```python
from build123d import *

# Parameters (mm, degrees)
SKETCH1_W            = 76
SKETCH1_H            = 41
BOSS_EXTRUDE1_DEPTH  = 1
SKETCH2_W            = 9
SKETCH2_H            = 9
BOSS_EXTRUDE2_DEPTH  = 1
SKETCH3_R            = 1.6
CUT_EXTRUDE1_DEPTH   = 1
FILLET1_R            = 1
FILLET3_R            = 3
FILLET1_OF_MIRROR2_R = 1
MIRROR3_OUTLINE_R    = 1.6
MIRROR3_DEPTH        = 1
FILLET4_R            = 3


# Read off the part's stored shape, not the designer's step: Mirror3
with BuildPart() as part:
    # Sketch1 → Boss-Extrude1 (new body)
    with BuildSketch(Plane(origin=(0, 0, 0), x_dir=(1, 0, 0), z_dir=(0, 1, 0))):
        Rectangle(SKETCH1_W, SKETCH1_H)
    boss_extrude1 = extrude(amount=BOSS_EXTRUDE1_DEPTH)

    # Sketch2 → Boss-Extrude2 (add)
    with BuildSketch(Plane(origin=(0, 1, 0), x_dir=(1, 0, 0), z_dir=(0, 1, 0))):
        with Locations((40.5, 23)):
            Rectangle(SKETCH2_W, SKETCH2_H)
    boss_extrude2 = extrude(amount=-BOSS_EXTRUDE2_DEPTH)

    # Sketch3 → Cut-Extrude1 (cut)
    with BuildSketch(Plane(origin=(0, 1, 0), x_dir=(1, 0, 0), z_dir=(0, 1, 0))):
        with Locations(Location((40.5, 22.887482194, 0), (0, 0, 270))):
            Circle(SKETCH3_R)
    cut_extrude1 = extrude(amount=-CUT_EXTRUDE1_DEPTH, mode=Mode.SUBTRACT)

    # Fillet1
    fillet1_edges = [part.edges().sort_by_distance(p)[0] for p in [
        (45, 0.5, -18.5),
        (36, 0.5, -27.5),
        (45, 0.5, -27.5),
    ]]
    fillet(fillet1_edges, radius=FILLET1_R)

    # Fillet3
    fillet3_edges = [part.edges().sort_by_distance(p)[0] for p in [
        (36, 0.5, -20.5),
        (38, 0.5, -18.5),
    ]]
    fillet(fillet3_edges, radius=FILLET3_R)

    # Mirror2: Boss-Extrude1, Boss-Extrude2, Cut-Extrude1 across plane
    add(boss_extrude1.mirror(Plane.XY))
    add(boss_extrude2.mirror(Plane.XY))
    add(cut_extrude1.mirror(Plane.XY), mode=Mode.SUBTRACT)

    # Fillet1 of Mirror2
    fillet1_of_mirror2_edges = [part.edges().sort_by_distance(p)[0] for p in [
        (45, 0.5, 18.5),
        (36, 0.5, 27.5),
        (45, 0.5, 27.5),
    ]]
    fillet(fillet1_of_mirror2_edges, radius=FILLET1_OF_MIRROR2_R)

    # Mirror3 outline → Mirror3 (add)
    # profile 1 of 2: a face of its own
    with BuildSketch(Plane(origin=(0, 0, 0), x_dir=(1, 0, 0), z_dir=(0, 1, 0))):
        with BuildLine():
            Line((-38, -20.5), (-38, -18.5))
            Line((-38, -18.5), (-44, -18.5))
            ThreePointArc((-44, -18.5), (-44.707106781, -18.792893219), (-45, -19.5))
            Line((-45, -19.5), (-45, -26.5))
            ThreePointArc((-45, -26.5), (-44.707106781, -27.207106781), (-44, -27.5))
            Line((-44, -27.5), (-37, -27.5))
            ThreePointArc((-37, -27.5), (-36.292893219, -27.207106781), (-36, -26.5))
            Line((-36, -26.5), (-36, -20.5))
            Line((-36, -20.5), (-38, -20.5))
        make_face()
        with Locations((-40.5, -22.887482194)):
            Circle(MIRROR3_OUTLINE_R, mode=Mode.SUBTRACT)
    # profile 2 of 2: a face of its own
    with BuildSketch(Plane(origin=(0, 0, 0), x_dir=(1, 0, 0), z_dir=(0, 1, 0))):
        with BuildLine():
            Line((-44, 18.5), (-38, 18.5))
            Line((-38, 18.5), (-38, 20.5))
            Line((-38, 20.5), (-36, 20.5))
            Line((-36, 20.5), (-36, 26.5))
            ThreePointArc((-36, 26.5), (-36.292893219, 27.207106781), (-37, 27.5))
            Line((-37, 27.5), (-44, 27.5))
            ThreePointArc((-44, 27.5), (-44.707106781, 27.207106781), (-45, 26.5))
            Line((-45, 26.5), (-45, 19.5))
            ThreePointArc((-45, 19.5), (-44.707106781, 18.792893219), (-44, 18.5))
        make_face()
        with Locations((-40.5, 22.887482194)):
            Circle(MIRROR3_OUTLINE_R, mode=Mode.SUBTRACT)
    extrude(amount=MIRROR3_DEPTH)

    # Fillet4
    fillet4_edges = [part.edges().sort_by_distance(p)[0] for p in [
        (-36, 0.5, 20.5),
        (-38, 0.5, 18.5),
        (-36, 0.5, -20.5),
        (-38, 0.5, -18.5),
        (36, 0.5, 20.5),
        (38, 0.5, 18.5),
    ]]
    fillet(fillet4_edges, radius=FILLET4_R)


solid = part.part
```
Input: part model. Units: mm. Frame: model coordinates. A direction names the side the tool comes from. Round coordinates to 2 decimals unless told otherwise and drop trailing zeros. Loops run counter-clockwise (first coordinate to the right, second up) from the corner with the lowest first, then second, coordinate; pieces in that order, holes last. Notation, with made-up numbers: (12.25, 54) -> (47.25, 54) arc R15 ccw to (47.25, 76) -> close; hole circle Ø4 at (22.5, -10). An arc over 180 degrees is marked (long way). Use one line per item in the form item = value. Start each with the question number.
Item 1: Set-up query: faces 1 (the face through (-35.1, 0.51, -21.36)), 2 (the face through (-35.14, 0.51, 21.4)), 3 (the face through (-38.9, 0.51, 17.64)), 4 (the face through (38.86, 0.51, -17.6)). Return all of +Z, -Z, +X, -X, +Y, -Y with unobstructed straight access to the full face (end or side cutting, diameter ignored); none if empty.
Item 2: Section query A-A on z = -6. Return the cut outline in (x, y).
Item 3: Section query B-B on x = -4.5. Return the cut outline in (y, z).
Item 4: Contact query for a flat-ended pin moving along its axis: pin 1 Ø0.5 at (y, z) = (0.5, 5.5) entering from +X. Output: stop coordinate, or through.
Item 5: Material intervals for L1, parallel to Z at x = -40.5, y = 0.25; L2, parallel to X at y = 0.7, z = 23; L3, parallel to X at y = 0.75, z = -7.5, sorted ascending. Write a range as from..to.
Item 6: Section query C-C on y = 0.25. Count the separate pieces of the cut face and the enclosed holes in it, then the cut area to 3 significant figures.
Item 7: Mould query, pull axis X, two halves, no side actions, for faces 5 (the face through (-40.847, 0.493, -21.326)), 6 (the face through (38.9, 0.51, 17.64)), 7 (the face through (-1, 1, 0)). Classes: pulls with the +X half, pulls with the -X half, needs draft (parallel to the pull), parting line crosses it, or undercut.
Ans:
q1.face_1 = -Z, +Y, -Y
q1.face_2 = +Z, +Y, -Y
q1.face_3 = -X, +Y, -Y
q1.face_4 = +X, +Y, -Y
q2.outline = (-38, 0) -> (38, 0) -> (38, 1) -> (-38, 1) -> close
q3.outline = (0, -20.5) -> (1, -20.5) -> (1, 20.5) -> (0, 20.5) -> close
q4.pin_1 = 38
q5.L1 = -27.5..-24.49, -21.29..-18.46, 18.46..21.29, 24.49..27.5
q5.L2 = -45..-42.1, -38.9..-35.96, 35.96..38.9, 42.1..45
q5.L3 = -38..38
q6.separate_pieces = 1
q6.enclosed_holes = 4
q6.area = 3,400 mm^2
q7.face_5 = undercut
q7.face_6 = pulls with the +X half
q7.face_7 = needs draft
